Check sheet for the modelled part. Datum: model origin and axes. Units: mm. A direction names the side the tool comes from. Coordinates: 2 decimals unless noted, no trailing zeros. Write each loop counter-clockwise with the first axis right and the second up, starting at its lowest first coordinate (ties: lowest second). Pieces come first, ordered by that corner, then holes. Notation, with made-up numbers: (21.25, -39.75) - (49.25, -39.75) arc R19 ccw to (49.25, -31.75) - close; hole circle Ø7 at (50.5, -12.5). An arc over 180 degrees is marked (long way). Use one line per item in the form item = value. Start each with the question number.
1. Cross-section at B-B on y = 1. Record the boundary of the cut face in (x, z) (3 decimals).
2. Draft check along Y on faces 1 (the face through (-62, -29.375, 2)), 2 (the face through (-1, 1, 0)), 3 (the face through (-5.38, -0.05, 1.97)). Enter one of: +Y half, -Y half, draft (parallel to the pull), parting line (faces both ways), or undercut.
3. Tool access check on faces 4 (the face through (-37, 31.875, 2)), 5 (the face through (-58, -13.275, 2)), 6 (the face through (52.5, -12, 2)). Record the directions out of +Z, -Z, +X, -X, +Y, -Y that give a thin tool (end or side, any length) a straight path to the whole face; none if there is none.
4. Cross-section at D-D on z = 1.05. Give the number of separate pieces and of enclosed holes in the cut face, then the cut area to 3 significant figures.
5. Scan lines: line 1 along Y through (x, z) = (-50, 2.7) (3 decimals); line 2 along Y through (x, z) = (-26.5, 1.45) (3 decimals); line 3 along X through (y, z) = (0, 3.2) (3 decimals). Record each from-to range of solid material in increasing order.
6. Cross-section at A-A on x = 50. Record the boundary of the cut face in (y, z) (3 decimals).
7. Cross-section at C-C on y = 20. Record the boundary of the cut face in (x, z).
8. Go/stop test with flat-tipped pins: pin 1 Ø1.2 at (y, z) = (-31, 2.5) entering from -X; pin 2 Ø0.5 at (y, z) = (-31.5, 3.5) entering from +X; pin 3 Ø1.2 at (x, z) = (-62, 2.5) entering from -Y (3 decimals). Record where each tip stops, or that it passes through.
```python
from build123d import *

# Parameters (mm, degrees)
SKETCH_1_W          = 120
SKETCH_1_H          = 83.75
SKETCH_1_W_2        = 4
SKETCH_1_H_2        = 11.25
EXTRUDE_1_DEPTH     = 4
SKETCH_2_W          = 7.5
SKETCH_2_H          = 2.8
SKETCH_2_W_2        = 2
SKETCH_2_H_2        = 5
CUT_EXTRUDE_1_DEPTH = 4
SKETCH_3_W          = 3
SKETCH_3_H          = 63.75
SKETCH_3_R          = 1.5
CUT_EXTRUDE_2_DEPTH = 77.586654353
FILLET_1_R          = 5
SKETCH_4_W          = 6
SKETCH_4_H          = 2
SKETCH_4_W_2        = 2
SKETCH_4_H_2        = 6
CUT_EXTRUDE_3_DEPTH = 1


with BuildPart() as part:
    # Эскиз1 → Бобышка-Вытянуть1 (new body)
    with BuildSketch(Plane.XY):
        Rectangle(SKETCH_1_W, SKETCH_1_H)
        with Locations((-62, -23.75)):
            Rectangle(SKETCH_1_W_2, SKETCH_1_H_2)
        with Locations((-62, 23.75)):
            Rectangle(SKETCH_1_W_2, SKETCH_1_H_2)
        with Locations((62, 23.75)):
            Rectangle(SKETCH_1_W_2, SKETCH_1_H_2)
        with Locations((62, -23.75)):
            Rectangle(SKETCH_1_W_2, SKETCH_1_H_2)
        with Locations((-62, 0)):
            Rectangle(SKETCH_1_W_2, SKETCH_1_H_2)
        with Locations((62, 0)):
            Rectangle(SKETCH_1_W_2, SKETCH_1_H_2)
    extrude(amount=EXTRUDE_1_DEPTH)

    # Эскиз2 → Вырез-Вытянуть1 (cut)
    with BuildSketch(Plane.XY.offset(4)):
        with Locations((-56.25, 35.625)):
            Rectangle(SKETCH_2_W, SKETCH_2_H)
        with Locations((-55, 35.625)):
            Rectangle(SKETCH_2_W_2, SKETCH_2_H_2)
        with Locations((-55, -35.625)):
            Rectangle(SKETCH_2_W_2, SKETCH_2_H_2)
        with Locations((-56.25, -35.625)):
            Rectangle(SKETCH_2_W, SKETCH_2_H)
        with Locations((-56.25, -11.875)):
            Rectangle(SKETCH_2_W, SKETCH_2_H)
        with Locations((-55, -11.875)):
            Rectangle(SKETCH_2_W_2, SKETCH_2_H_2)
        with Locations((55, -11.875)):
            Rectangle(SKETCH_2_W_2, SKETCH_2_H_2)
        with Locations((56.25, -11.875)):
            Rectangle(SKETCH_2_W, SKETCH_2_H)
        with Locations((56.25, -35.625)):
            Rectangle(SKETCH_2_W, SKETCH_2_H)
        with Locations((55, -35.625)):
            Rectangle(SKETCH_2_W_2, SKETCH_2_H_2)
        with Locations((55, 35.625)):
            Rectangle(SKETCH_2_W_2, SKETCH_2_H_2)
        with Locations((56.25, 35.625)):
            Rectangle(SKETCH_2_W, SKETCH_2_H)
    extrude(amount=-CUT_EXTRUDE_1_DEPTH, mode=Mode.SUBTRACT)

    # Эскиз3 → Вырез-Вытянуть2 (cut, through all)
    with BuildSketch(Plane.XY.offset(4)):
        with Locations((-36.5, 0)):
            Rectangle(SKETCH_3_W, SKETCH_3_H)
        with Locations((36.5, 0)):
            Rectangle(SKETCH_3_W, SKETCH_3_H)
        Polygon((-25.125, 22.645469736), (-25.125, -22.645469736), (-3.459853629, 0), align=None)
        Polygon((21.773371479, 26.375), (-21.773371479, 26.375), (0, 3.616408092), align=None)
        Polygon((21.773371479, -26.375), (0, -3.616408092), (-21.773371479, -26.375), align=None)
        Polygon((25.125, -22.645469736), (25.125, 22.645469736), (3.459853629, 0), align=None)
        with Locations((-27.625, 28.875)):
            Circle(SKETCH_3_R)
        with Locations((27.625, 28.875)):
            Circle(SKETCH_3_R)
        with Locations((27.625, -28.875)):
            Circle(SKETCH_3_R)
        with Locations((-27.625, -28.875)):
            Circle(SKETCH_3_R)
        with Locations((50, -23.75)):
            Circle(SKETCH_3_R)
        with Locations(Location((50, 23.75, 0), (0, 0, 180))):
            Circle(SKETCH_3_R)
        with Locations((-50, 23.75)):
            Circle(SKETCH_3_R)
        with Locations(Location((-50, -23.75, 0), (0, 0, 180))):
            Circle(SKETCH_3_R)
    extrude(amount=-CUT_EXTRUDE_2_DEPTH, mode=Mode.SUBTRACT)

    # Скругление1
    fillet_1_edges = [part.edges().sort_by_distance(p)[0] for p in [
        (-21.773371479, -26.375, 2),
        (0, -3.616408092, 2),
        (21.773371479, -26.375, 2),
        (-3.459853629, 0, 2),
        (-25.125, -22.645469736, 2),
        (-25.125, 22.645469736, 2),
        (25.125, -22.645469736, 2),
        (3.459853629, 0, 2),
        (25.125, 22.645469736, 2),
        (0, 3.616408092, 2),
        (-21.773371479, 26.375, 2),
        (21.773371479, 26.375, 2),
    ]]
    fillet(fillet_1_edges, radius=FILLET_1_R)

    # Эскиз4 → Вырез-Вытянуть3 (cut)
    with BuildSketch(Plane.XY.offset(4)):
        with Locations((-43.625, 9.625)):
            Rectangle(SKETCH_4_W, SKETCH_4_H)
        with Locations((-43.625, 28.875)):
            Rectangle(SKETCH_4_W, SKETCH_4_H)
        with Locations((-43.625, 28.875)):
            Rectangle(SKETCH_4_W_2, SKETCH_4_H_2)
        with Locations((-43.625, -9.625)):
            Rectangle(SKETCH_4_W, SKETCH_4_H)
        with Locations((-43.625, -9.625)):
            Rectangle(SKETCH_4_W_2, SKETCH_4_H_2)
        with Locations((-43.625, -28.875)):
            Rectangle(SKETCH_4_W, SKETCH_4_H)
        with Locations((43.625, -28.875)):
            Rectangle(SKETCH_4_W_2, SKETCH_4_H_2)
        with Locations((43.625, -28.875)):
            Rectangle(SKETCH_4_W, SKETCH_4_H)
        with Locations((43.625, -9.625)):
            Rectangle(SKETCH_4_W, SKETCH_4_H)
        with Locations((43.625, 9.625)):
            Rectangle(SKETCH_4_W_2, SKETCH_4_H_2)
        with Locations((43.625, 9.625)):
            Rectangle(SKETCH_4_W, SKETCH_4_H)
        with Locations((43.625, 28.875)):
            Rectangle(SKETCH_4_W, SKETCH_4_H)
    extrude(amount=-CUT_EXTRUDE_3_DEPTH, mode=Mode.SUBTRACT)


solid = part.part
```
Final values:
q1.outline = (-64, 0) - (-38, 0) - (-38, 4) - (-64, 4) - close; (-35, 0) - (-25.125, 0) - (-25.125, 4) - (-35, 4) - close; (-5.481, 0) - (5.481, 0) - (5.481, 4) - (-5.481, 4) - close; (25.125, 0) - (35, 0) - (35, 4) - (25.125, 4) - close; (38, 0) - (64, 0) - (64, 4) - (38, 4) - close
q2.face_1 = -Y half
q2.face_2 = draft
q2.face_3 = undercut
q3.face_4 = +Z, -Z
q3.face_5 = +Z, -Z, -X
q3.face_6 = +Z, -Z, +X
q4.separate_pieces = 1
q4.enclosed_holes = 14
q4.area = 8,030 mm²
q5.line_1 = -41.875 to -25.25, -22.25 to 22.25, 25.25 to 41.875
q5.line_2 = -41.875 to -29.867, -27.883 to 27.883, 29.867 to 41.875
q5.line_3 = -64 to -38, -35 to -25.125, -5.38 to 5.38, 25.125 to 35, 38 to 64
q6.outline = (-41.875, 0) - (-25.25, 0) - (-25.25, 4) - (-41.875, 4) - close; (-22.25, 0) - (22.25, 0) - (22.25, 4) - (-22.25, 4) - close; (25.25, 0) - (41.875, 0) - (41.875, 4) - (25.25, 4) - close
q7.outline = (-64, 0) - (-38, 0) - (-38, 4) - (-64, 4) - close; (-35, 0) - (-14.88, 0) - (-14.88, 4) - (-35, 4) - close; (14.88, 0) - (35, 0) - (35, 4) - (14.88, 4) - close; (38, 0) - (64, 0) - (64, 4) - (38, 4) - close
q8.pin_1 = -60
q8.pin_2 = 60
q8.pin_3 = -29.375
